Answer from the drawing. Dimensions are ordinates in mm from the lowest x, y and z of the part. Give positions to 0.01 mm unless a question says otherwise; leave off trailing zeros. Order: outer loops, then holes, each group sorted by start corner. A loop starts at its lowest first (then second) coordinate and runs counter-clockwise, first axis right, second up. Notation, with made-up numbers: (38, 23.5) - (75, 23.5) arc R11 cw to (75, 39.5) - close; hole circle Ø11 at (32, 63). An arc over 180 degrees is marked (long way). One line per item, written item: value. Start each with the question number.
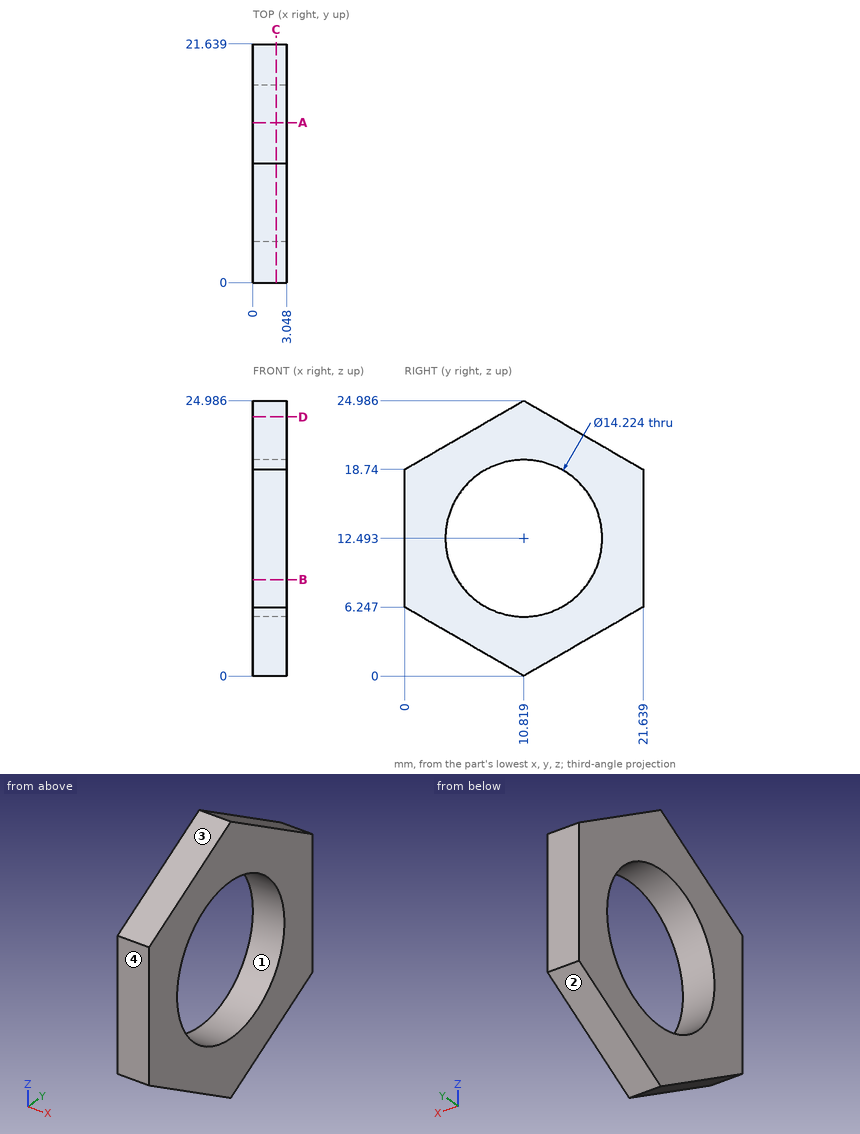
1) Section A-A on y = 14.5 is taken. Write down the section's boundary in (x, z) (1 decimal).
2) The mould has two halves that part along Z. Classify the marked faces 1, 2, 3 and 4: +Z half, -Z half, draft (parallel to the pull), parting line (faces both ways), or undercut.
3) This flat-tipped pin is pushed along its axis until it touches: pin 1 (11.5 mm diameter, centred on y = 10.82, z = 12.49, fed in from -X). Where does it stop, or does it pass through?
4) Section D-D on z = 23.5 is taken. Write down the section's boundary in (x, y) (1 decimal).
5) Section B-B on z = 8.75 is taken. Write down the section's boundary in (x, y).
6) Find the intervals of material crossed by probe 1 along Y at (x, z) = (2.9, 12.75); probe 2 along Z at (x, y) = (0.85, 16.75) (1 decimal); probe 3 along Z at (x, y) = (2.65, 11) (1 decimal), in increasing order. Write a range as from..to.
7) Section C-C on x = 2.1 is taken. Write down the section's boundary in (y, z).
Solved:
1. outline: (0, 2.1) - (3, 2.1) - (3, 6.4) - (0, 6.4) - close; (0, 18.6) - (3, 18.6) - (3, 22.9) - (0, 22.9) - close
2. face 1: undercut
2. face 2: -Z half
2. face 3: +Z half
2. face 4: draft
3. pin 1: passes through
4. outline: (0, 8.2) - (3, 8.2) - (3, 13.4) - (0, 13.4) - close
5. outline: (0, 0) - (3.05, 0) - (3.05, 4.77) - (0, 4.77) - close; (0, 16.87) - (3.05, 16.87) - (3.05, 21.64) - (0, 21.64) - close
6. probe 1: y = 0..3.71, 17.93..21.64
6. probe 2: z = 3.4..8.6, 16.4..21.6
6. probe 3: z = 0.1..5.4, 19.6..24.9
7. outline: (0, 6.25) - (10.82, 0) - (21.64, 6.25) - (21.64, 18.74) - (10.82, 24.99) - (0, 18.74) - close; hole circle Ø14.22 at (10.82, 12.49)
